Autodesk Inventor part; units mm, degrees
ref_plane "YZ Plane" through (0, 0, 0) normal (1, 0, 0) x (0, 1, 0)
ref_plane "XZ Plane" through (0, 0, 0) normal (0, 1, 0) x (-1, 0, 0)
ref_plane "XY Plane" through (0, 0, 0) normal (0, 0, 1) x (1, 0, 0)
sketch "Sketch1" plane through (0, 0, 0) normal (0, 1, 0) x (-1, 0, 0)
  circle A0 centre (0, 0) radius 26.05
  dimension "d0" = 52.1
extrude "Extrusion1" add sketch "Sketch1" along normal blind 100.6
sketch "Sketch2" plane through (0, 100.6, 0) normal (0, 1, 0) x (1, 0, 0)
  circle A0 centre (0, 0) radius 10
  dimension "d3" = 20
extrude "Extrusion2" add sketch "Sketch2" along normal blind 4.6
sketch "Sketch3" plane through (0, 105.2, 0) normal (0, 1, 0) x (1, 0, 0)
  circle A0 centre (0, 0) radius 10
  circle A1 centre (0, 0) radius 26.05
extrude "Extrusion3" add sketch "Sketch3" along normal blind 26 contours A0 | A1
sketch "Sketch4" plane through (0, 0, 0) normal (0, -1, 0) x (1, 0, 0)
  circle A0 centre (0, 0) radius 9.5
  dimension "d8" = 19
extrude "Extrusion4" add sketch "Sketch4" along normal blind 50
properties part number "SPINDLE"
Source: CAD feature listing. Evaluate the final solid. Frame: model axes, mm. A direction names the side the tool comes from. Coordinates: 2 decimals unless noted, no trailing zeros. Loops run counter-clockwise (first coordinate to the right, second up) from the corner with the lowest first, then second, coordinate; pieces in that order, holes last. Notation, with made-up numbers: (-40, -33) - (-7, -33) arc R16 cw to (-7, -8) - close; hole circle Ø4 at (86.5, 28.5). An arc over 180 degrees is marked (long way). One line per item, written item: value. Start each with the question number.
1. Ray query, L1, parallel to Y at x = -19.5, z = -7; L2, parallel to X at y = 84.5, z = 1; L3, parallel to X at y = -30, z = 4. Return the intervals inside material, ascending.
2. Section D-D (x = -18). Return the cut outline in (y, z).
3. Section C-C (z = 0). Return the cut outline in (x, y).
4. Mould query, pull axis Y, two halves, no side actions, for faces 4 (the cylindrical face through (-2.17, 102.87, -9.76)), 5 (the flat face through (-11, 100.6, 0)), 6 (the cylindrical face through (20.672, 49.596, 15.851)), 7 (the flat face through (0, -50, 0)). Classes: pulls with the +Y half, pulls with the -Y half, needs draft (parallel to the pull), parting line crosses it, or undercut.
5. Set-up query: faces 1 (the cylindrical face through (4.38, -24.65, 8.43)), 2 (the flat face through (11, 105.2, 0)), 3 (the flat face through (0, 131.2, 0)). Return all of +Z, -Z, +X, -X, +Y, -Y with unobstructed straight access to the full face (end or side cutting, diameter ignored); none if empty.
6. Section B-B (x = 0). Return the cut outline in (y, z), and give its area (3 significant figures).
7. Section A-A (z = 22). Return the cut outline in (x, y), and give its area (3 significant figures).
8. Contact query for flat-ended pins moving along their axis: P1, Ø10, axis at x = 19.5, y = 78.5, coming from the -Z side; P2, Ø8, axis at x = -19.5, z = -1.5, coming from the -Y side; P3, Ø6, axis at y = 76.5, z = 12, coming from the +X side. Output: stop coordinate, or through.
Verdict:
1. L1: y = 0 to 100.6, 105.2 to 131.2
1. L2: x = -26.03 to 26.03
1. L3: x = -8.62 to 8.62
2. outline: (0, -18.83) - (100.6, -18.83) - (100.6, 18.83) - (0, 18.83) - close; (105.2, -18.83) - (131.2, -18.83) - (131.2, 18.83) - (105.2, 18.83) - close
3. outline: (-26.05, 0) - (-9.5, 0) - (-9.5, -50) - (9.5, -50) - (9.5, 0) - (26.05, 0) - (26.05, 100.6) - (10, 100.6) - (10, 105.2) - (26.05, 105.2) - (26.05, 131.2) - (-26.05, 131.2) - (-26.05, 105.2) - (-10, 105.2) - (-10, 100.6) - (-26.05, 100.6) - close
4. face 4: undercut
4. face 5: undercut
4. face 6: needs draft
4. face 7: pulls with the -Y half
5. face 1: -Y
5. face 2: none
5. face 3: +Z, -Z, +X, -X, +Y
6. outline: (-50, -9.5) - (0, -9.5) - (0, -26.05) - (100.6, -26.05) - (100.6, -10) - (105.2, -10) - (105.2, -26.05) - (131.2, -26.05) - (131.2, 26.05) - (105.2, 26.05) - (105.2, 10) - (100.6, 10) - (100.6, 26.05) - (0, 26.05) - (0, 9.5) - (-50, 9.5) - close
6. area: 7,640 mm2
7. outline: (-13.95, 0) - (13.95, 0) - (13.95, 100.6) - (-13.95, 100.6) - close; (-13.95, 105.2) - (13.95, 105.2) - (13.95, 131.2) - (-13.95, 131.2) - close
7. area: 3,530 mm2
8. P1: stops at z = -21.64
8. P2: stops at y = 0
8. P3: stops at x = 24.45
